Geometry: final body of the model. Coordinates: model frame, mm. Give positions to 0.01 mm unless a question says otherwise; leave off trailing zeros. One line per item, written item: value.
```python
from build123d import *

# Parameters (mm, degrees)
BOSS_EXTRUDE1_DEPTH   = 2016
SKETCH3_R             = 3.4
CUT_EXTRUDE1_DEPTH    = 2018.983151565
CUT_EXTRUDE2_DEPTH    = 2018.983151565
FILLET1_R             = 1
FILLET2_R             = 1
FILLET3_R             = 1
CUT_EXTRUDE3_DEPTH    = 2018.983151565
CUT_EXTRUDE4_DEPTH    = 2018.983151565
FILLET4_R             = 1
FILLET5_R             = 1
FILLET6_R             = 1
FILLET7_R             = 1
FILLET8_R             = 1
FILLET9_R             = 1
FILLET10_R            = 1
FILLET11_R            = 1
MIRROR11_COPY_1_DEPTH = 2018.983151565
MIRROR11_COPY_2_DEPTH = 2018.983151565
CUT_EXTRUDE5_DEPTH    = 1000


with BuildPart() as part:
    # Sketch1 → Boss-Extrude1 (new body)
    with BuildSketch(Plane(origin=(0, 0, 0), x_dir=(1, 0, 0), z_dir=(0, 1, 0))):
        with BuildLine():
            Line((5, 0), (75, 0))
            ThreePointArc((75, 0), (78.535533906, -1.464466094), (80, -5))
            Line((80, -5), (80, -35))
            ThreePointArc((80, -35), (78.535533906, -38.535533906), (75, -40))
            Line((75, -40), (5, -40))
            ThreePointArc((5, -40), (1.464466094, -38.535533906), (0, -35))
            Line((0, -35), (0, -5))
            ThreePointArc((0, -5), (1.464466094, -1.464466094), (5, 0))
        make_face()
    extrude(amount=BOSS_EXTRUDE1_DEPTH)

    # Sketch3 → Cut-Extrude1 (cut, through all)
    with BuildSketch(Plane(origin=(0, 2016, 0), x_dir=(1, 0, 0), z_dir=(0, 1, 0))):
        with Locations(Location((20, -20, 0), (0, 0, 270))):
            Circle(SKETCH3_R)
    cut_extrude1 = extrude(amount=-CUT_EXTRUDE1_DEPTH, mode=Mode.SUBTRACT)

    # Mirror3: Cut-Extrude1 across plane
    add(cut_extrude1.mirror(Plane(origin=(40, 0, 0), x_dir=(0, 0, 1), z_dir=(1, 0, 0))), mode=Mode.SUBTRACT)

    # Sketch7 → Cut-Extrude2 (cut, through all)
    with BuildSketch(Plane(origin=(0, 0, 0), x_dir=(-1, 0, 0), z_dir=(0, -1, 0))):
        with BuildLine():
            Line((-15.9, -40), (-24.1, -40))
            Line((-24.1, -40), (-24.1, -36.5))
            ThreePointArc((-24.1, -36.5), (-24.392893219, -35.792893219), (-25.1, -35.5))
            Line((-25.1, -35.5), (-29.489753594, -35.5))
            ThreePointArc((-29.489753594, -35.5), (-30.415270825, -34.8787055), (-30.190750526, -33.786835712))
            Line((-30.190750526, -33.786835712), (-24.391814382, -28.086835712))
            ThreePointArc((-24.391814382, -28.086835712), (-24.069522951, -27.874482769), (-23.69081745, -27.8))
            Line((-23.69081745, -27.8), (-16.309186536, -27.8))
            ThreePointArc((-16.309186536, -27.8), (-15.930477876, -27.874484063), (-15.608184734, -28.086840499))
            Line((-15.608184734, -28.086840499), (-9.809327805, -33.786840499))
            ThreePointArc((-9.809327805, -33.786840499), (-9.584813669, -34.87870866), (-10.510329607, -35.5))
            Line((-10.510329607, -35.5), (-14.9, -35.5))
            ThreePointArc((-14.9, -35.5), (-15.607106781, -35.792893219), (-15.9, -36.5))
            Line((-15.9, -36.5), (-15.9, -40))
        make_face()
    cut_extrude2 = extrude(amount=-CUT_EXTRUDE2_DEPTH, mode=Mode.SUBTRACT)

    # Fillet1
    fillet1_edges = [part.edges().sort_by_distance(p)[0] for p in [
        (15.9, 1008, 40),
        (24.1, 1008, 40),
    ]]
    fillet(fillet1_edges, radius=FILLET1_R)

    # Mirror8: Cut-Extrude2 across plane
    add(cut_extrude2.mirror(Plane(origin=(40, 0, 0), x_dir=(0, 0, 1), z_dir=(1, 0, 0))), mode=Mode.SUBTRACT)

    # Fillet2
    fillet2_edges = [part.edges().sort_by_distance(p)[0] for p in [
        (55.9, 1008, 40),
    ]]
    fillet(fillet2_edges, radius=FILLET2_R)

    # Fillet3
    fillet3_edges = [part.edges().sort_by_distance(p)[0] for p in [
        (64.1, 1008, 40),
    ]]
    fillet(fillet3_edges, radius=FILLET3_R)

    # Sketch9 → Cut-Extrude3 (cut, through all)
    with BuildSketch(Plane(origin=(0, 0, 0), x_dir=(1, 0, 0), z_dir=(0, 1, 0))):
        with BuildLine():
            Line((14.899846923, -4.500713815), (10.450461284, -4.500713815))
            ThreePointArc((10.450461284, -4.500713815), (9.526581751, -5.118030383), (9.743354502, -6.207820596))
            Line((9.743354502, -6.207820596), (15.442640687, -11.907106781))
            ThreePointArc((15.442640687, -11.907106781), (15.767064036, -12.123879533), (16.149747468, -12.2))
            Line((16.149747468, -12.2), (23.850252532, -12.2))
            ThreePointArc((23.850252532, -12.2), (24.232935964, -12.123879533), (24.557359313, -11.907106781))
            Line((24.557359313, -11.907106781), (30.257359313, -6.207106781))
            ThreePointArc((30.257359313, -6.207106781), (30.474132064, -5.117316568), (29.550252532, -4.5))
            Line((29.550252532, -4.5), (25.099846964, -4.5))
            ThreePointArc((25.099846964, -4.5), (24.392724723, -4.207091321), (24.099846965, -3.499956273))
            Line((24.099846965, -3.499956273), (24.100000008, 0))
            Line((24.100000008, 0), (15.9, 0))
            Line((15.9, 0), (15.899846922, -3.500757542))
            ThreePointArc((15.899846922, -3.500757542), (15.606938244, -4.207836056), (14.899846923, -4.500713815))
        make_face()
    cut_extrude3 = extrude(amount=CUT_EXTRUDE3_DEPTH, mode=Mode.SUBTRACT)

    # Mirror9: Cut-Extrude3 across plane
    add(cut_extrude3.mirror(Plane(origin=(40, 0, 0), x_dir=(0, 0, 1), z_dir=(1, 0, 0))), mode=Mode.SUBTRACT)

    # Sketch10 → Cut-Extrude4 (cut, through all)
    with BuildSketch(Plane(origin=(0, 0, 0), x_dir=(1, 0, 0), z_dir=(0, 1, 0))):
        with BuildLine():
            Line((4.5, -14.9), (4.5, -10.58605332))
            ThreePointArc((4.5, -10.58605332), (5.126159695, -9.658560233), (6.220486853, -9.892584724))
            Line((6.220486853, -9.892584724), (11.920486853, -15.814662646))
            ThreePointArc((11.920486853, -15.814662646), (12.127493087, -16.134290938), (12.2, -16.508131242))
            Line((12.2, -16.508131242), (12.2, -23.491868758))
            ThreePointArc((12.2, -23.491868758), (12.127493087, -23.865709062), (11.920486853, -24.185337354))
            Line((11.920486853, -24.185337354), (6.220486853, -30.107415276))
            ThreePointArc((6.220486853, -30.107415276), (5.126159695, -30.341439767), (4.5, -29.41394668))
            Line((4.5, -29.41394668), (4.5, -25.1))
            ThreePointArc((4.5, -25.1), (4.207106781, -24.392893219), (3.5, -24.1))
            Line((3.5, -24.1), (0, -24.1))
            Line((0, -24.1), (0, -15.9))
            Line((0, -15.9), (3.5, -15.9))
            ThreePointArc((3.5, -15.9), (4.207106781, -15.607106781), (4.5, -14.9))
        make_face()
    cut_extrude4 = extrude(amount=CUT_EXTRUDE4_DEPTH, mode=Mode.SUBTRACT)

    # Fillet4
    fillet4_edges = [part.edges().sort_by_distance(p)[0] for p in [
        (24.100000008, 1008, 0),
    ]]
    fillet(fillet4_edges, radius=FILLET4_R)

    # Fillet5
    fillet5_edges = [part.edges().sort_by_distance(p)[0] for p in [
        (64.1, 1008, 0),
    ]]
    fillet(fillet5_edges, radius=FILLET5_R)

    # Fillet6
    fillet6_edges = [part.edges().sort_by_distance(p)[0] for p in [
        (55.899999992, 1008, 0),
    ]]
    fillet(fillet6_edges, radius=FILLET6_R)

    # Fillet7
    fillet7_edges = [part.edges().sort_by_distance(p)[0] for p in [
        (15.9, 1008, 0),
    ]]
    fillet(fillet7_edges, radius=FILLET7_R)

    # Fillet8
    fillet8_edges = [part.edges().sort_by_distance(p)[0] for p in [
        (0, 1008, 24.1),
    ]]
    fillet(fillet8_edges, radius=FILLET8_R)

    # Fillet9
    fillet9_edges = [part.edges().sort_by_distance(p)[0] for p in [
        (0, 1008, 15.9),
    ]]
    fillet(fillet9_edges, radius=FILLET9_R)

    # Mirror10: Cut-Extrude4 across plane
    add(cut_extrude4.mirror(Plane(origin=(40, 0, 0), x_dir=(0, 0, 1), z_dir=(1, 0, 0))), mode=Mode.SUBTRACT)

    # Fillet10
    fillet10_edges = [part.edges().sort_by_distance(p)[0] for p in [
        (80, 1008, 15.9),
    ]]
    fillet(fillet10_edges, radius=FILLET10_R)

    # Fillet11
    fillet11_edges = [part.edges().sort_by_distance(p)[0] for p in [
        (80, 1008, 24.1),
    ]]
    fillet(fillet11_edges, radius=FILLET11_R)

    # Mirror11 copy 1 sketch → Mirror11 copy 1 (cut, through all)
    with BuildSketch(Plane(origin=(40, 0, 0), x_dir=(1, 0, 0), z_dir=(0, 1, 0))):
        with BuildLine():
            Line((4.5, -14.9), (4.5, -10.58605332))
            ThreePointArc((4.5, -10.58605332), (5.126159695, -9.658560233), (6.220486853, -9.892584724))
            Line((6.220486853, -9.892584724), (11.920486853, -15.814662646))
            ThreePointArc((11.920486853, -15.814662646), (12.127493087, -16.134290938), (12.2, -16.508131242))
            Line((12.2, -16.508131242), (12.2, -23.491868758))
            ThreePointArc((12.2, -23.491868758), (12.127493087, -23.865709062), (11.920486853, -24.185337354))
            Line((11.920486853, -24.185337354), (6.220486853, -30.107415276))
            ThreePointArc((6.220486853, -30.107415276), (5.126159695, -30.341439767), (4.5, -29.41394668))
            Line((4.5, -29.41394668), (4.5, -25.1))
            ThreePointArc((4.5, -25.1), (4.207106781, -24.392893219), (3.5, -24.1))
            Line((3.5, -24.1), (0, -24.1))
            Line((0, -24.1), (0, -15.9))
            Line((0, -15.9), (3.5, -15.9))
            ThreePointArc((3.5, -15.9), (4.207106781, -15.607106781), (4.5, -14.9))
        make_face()
    extrude(amount=MIRROR11_COPY_1_DEPTH, mode=Mode.SUBTRACT)

    # Mirror11 copy 2 sketch → Mirror11 copy 2 (cut, through all)
    with BuildSketch(Plane(origin=(120, 0, 0), x_dir=(-1, 0, 0), z_dir=(0, 1, 0))):
        with BuildLine():
            Line((4.5, 14.9), (4.5, 10.58605332))
            ThreePointArc((4.5, 10.58605332), (5.126159695, 9.658560233), (6.220486853, 9.892584724))
            Line((6.220486853, 9.892584724), (11.920486853, 15.814662646))
            ThreePointArc((11.920486853, 15.814662646), (12.127493087, 16.134290938), (12.2, 16.508131242))
            Line((12.2, 16.508131242), (12.2, 23.491868758))
            ThreePointArc((12.2, 23.491868758), (12.127493087, 23.865709062), (11.920486853, 24.185337354))
            Line((11.920486853, 24.185337354), (6.220486853, 30.107415276))
            ThreePointArc((6.220486853, 30.107415276), (5.126159695, 30.341439767), (4.5, 29.41394668))
            Line((4.5, 29.41394668), (4.5, 25.1))
            ThreePointArc((4.5, 25.1), (4.207106781, 24.392893219), (3.5, 24.1))
            Line((3.5, 24.1), (0, 24.1))
            Line((0, 24.1), (0, 15.9))
            Line((0, 15.9), (3.5, 15.9))
            ThreePointArc((3.5, 15.9), (4.207106781, 15.607106781), (4.5, 14.9))
        make_face()
    extrude(amount=MIRROR11_COPY_2_DEPTH, mode=Mode.SUBTRACT)

    # Mirror12: Cut-Extrude4 across plane
    add(cut_extrude4.mirror(Plane.ZY.offset(-20)), mode=Mode.SUBTRACT)

    # Sketch12 → Cut-Extrude5 (cut)
    with BuildSketch(Plane(origin=(0, 0, 0), x_dir=(-1, 0, 0), z_dir=(0, -1, 0))):
        with BuildLine():
            Line((-28.079513147, -24.185337354), (-39.327067998, -35.871108628))
            ThreePointArc((-39.327067998, -35.871108628), (-40.049082116, -36.177638866), (-40.770156561, -35.868904648))
            Line((-40.770156561, -35.868904648), (-51.922601709, -24.210885791))
            ThreePointArc((-51.922601709, -24.210885791), (-52.128062958, -23.892044517), (-52.2, -23.519621175))
            Line((-52.2, -23.519621175), (-52.2, -16.508131242))
            ThreePointArc((-52.2, -16.508131242), (-52.127493087, -16.134290938), (-51.920486853, -15.814662646))
            Line((-51.920486853, -15.814662646), (-40.720486853, -4.17829901))
            ThreePointArc((-40.720486853, -4.17829901), (-40, -3.871767606), (-39.279513147, -4.17829901))
            Line((-39.279513147, -4.17829901), (-28.079513147, -15.814662646))
            ThreePointArc((-28.079513147, -15.814662646), (-27.872506913, -16.134290938), (-27.8, -16.508131242))
            Line((-27.8, -16.508131242), (-27.8, -23.491868758))
            ThreePointArc((-27.8, -23.491868758), (-27.872506913, -23.865709062), (-28.079513147, -24.185337354))
        make_face()
    extrude(amount=-CUT_EXTRUDE5_DEPTH, mode=Mode.SUBTRACT)


solid = part.part
```
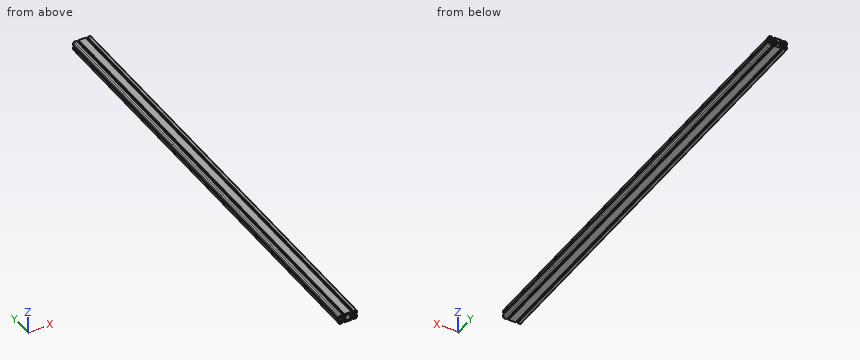
1) First-contact query: pin 1 (1.2 mm diameter, centred on y = 806.5, z = 37.5, fed in from -X); pin 2 (2 mm diameter, centred on y = 998, z = 21.5, fed in from -X); pin 3 (3 mm diameter, centred on x = 3, y = 1411, fed in from +Z). Flat tips, straight axial feed; report the tip coordinate or a pass-through.
Answers below:
pin 1: x = 0.38
pin 2: x = 12.2
pin 3: z = 39.97
2) Section A-A, the plane y = 648.5. Count the separate pieces of the cut face and the enclosed holes in it, then the cut area to 3 significant figures.
Answers below:
separate pieces: 1
enclosed holes: 3
area: 1,660 mm^2
3) Material intervals for line 1 along X through (y, z) = (1511, 34.5); line 2 along X through (y, z) = (1611, 20); line 3 along X through (y, z) = (1444, 6.5), sorted ascending.
Answers below:
line 1: 0 to 9.51, 30.49 to 49.51, 70.49 to 80
line 2: 12.2 to 16.6, 23.4 to 27.8, 52.2 to 56.6, 63.4 to 67.8
line 3: 0 to 10.04, 29.96 to 50.04, 69.96 to 80
